Source: three-view drawing plus pictorial views. Frame: mm from the lowest corner of the part. Coordinates: 2 decimals unless noted, no trailing zeros. Write each loop counter-clockwise with the first axis right and the second up, starting at its lowest first coordinate (ties: lowest second). Pieces come first, ordered by that corner, then holes. Notation, with made-up numbers: (-11, 46) -> (-1, 46) arc R11 ccw to (-1, 60) -> close; hole circle Ø8 at (21.25, 51). An arc over 180 degrees is marked (long way). One line per item, written item: value. Start each with the question number.
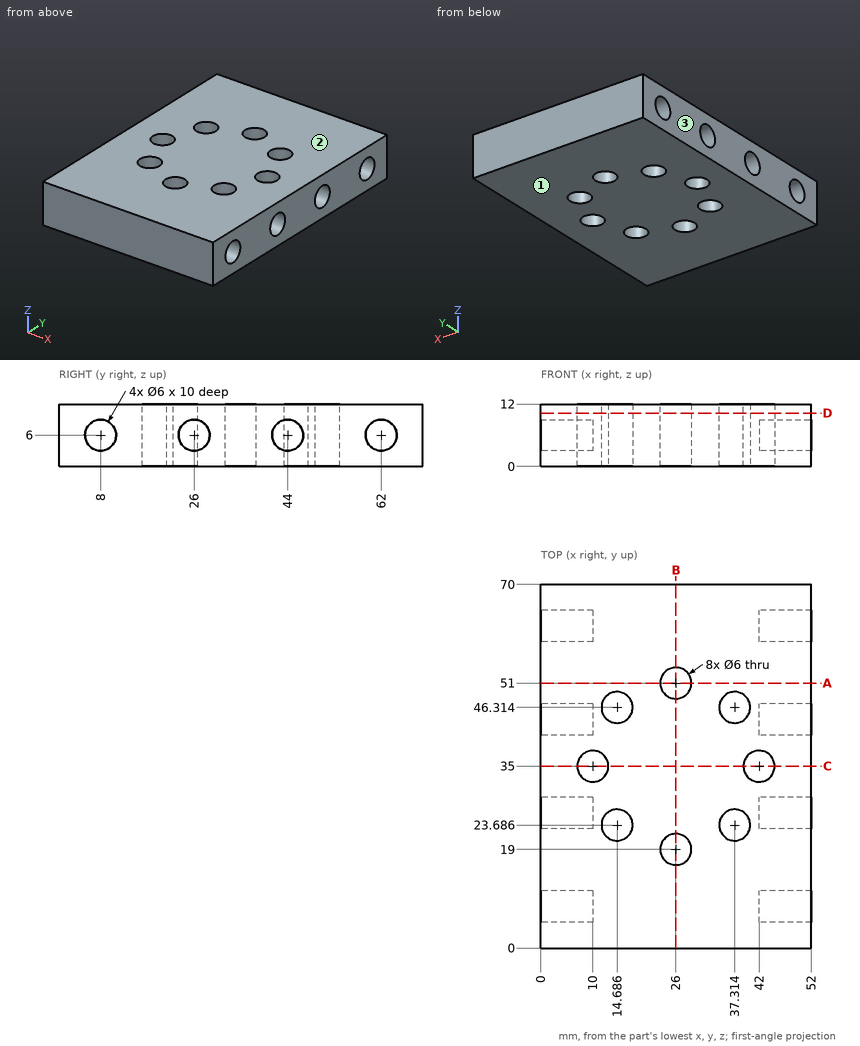
Q1. Draft query along Z for the marked faces 1, 2 and 3. Return one class per face: pulls with the +Z half, pulls with the -Z half, needs draft (parallel to the pull), parting line crosses it, or undercut.
Q2. Cut plane D-D on z = 10.25. Count the separate pieces of the cut face and the enclosed holes in it, and give its area (3 significant figures).
Q3. Line query: L1, parallel to Y at x = 15, z = 11; L2, parallel to Y at x = 2.75, z = 6; L3, parallel to Y at x = 26, z = 5.5. Output: solid intervals per line, ascending. Write a range as from..to.
Q4. Cut plane B-B on x = 26. Output: boundary loops of the cut face in (y, z).
Q5. First-contact query: P1, Ø3.5, axis at y = 8, z = 6, coming from the +X side; P2, Ø5.5, axis at y = 8, z = 6, coming from the -X side. Flat tips, straight axial feed; report the tip coordinate or a pass-through.
Q6. Cut plane A-A on y = 51. Output: boundary loops of the cut face in (x, z), and give its area (3 significant figures).
Q7. Cut plane C-C on y = 35. Output: boundary loops of the cut face in (x, z), and give its area (3 significant figures).
Solution:
1. face 1: pulls with the -Z half
1. face 2: pulls with the +Z half
1. face 3: needs draft
2. separate pieces: 1
2. enclosed holes: 8
2. area: 3,410 mm²
3. L1: 0..20.7, 26.67..43.33, 49.3..70
3. L2: 0..5, 11..23, 29..41, 47..59, 65..70
3. L3: 0..16, 22..48, 54..70
4. outline: (0, 0) -> (16, 0) -> (16, 12) -> (0, 12) -> close; (22, 0) -> (48, 0) -> (48, 12) -> (22, 12) -> close; (54, 0) -> (70, 0) -> (70, 12) -> (54, 12) -> close
5. P1: x = 42
5. P2: x = 10
6. outline: (0, 0) -> (23, 0) -> (23, 12) -> (0, 12) -> close; (29, 0) -> (52, 0) -> (52, 12) -> (29, 12) -> close
6. area: 552 mm²
7. outline: (0, 0) -> (7, 0) -> (7, 12) -> (0, 12) -> close; (13, 0) -> (39, 0) -> (39, 12) -> (13, 12) -> close; (45, 0) -> (52, 0) -> (52, 12) -> (45, 12) -> close
7. area: 480 mm²
